Input: part model. Units: mm. Frame: model coordinates. Round coordinates to 2 decimals unless told otherwise and drop trailing zeros. Write each loop counter-clockwise with the first axis right and the second up, starting at its lowest first coordinate (ties: lowest second). Pieces come first, ordered by that corner, then holes. Notation, with made-up numbers: (27.5, 8.5) -> (35.5, 8.5) arc R17 cw to (35.5, 17.5) -> close; hole circle Ø9 at (39.25, 76.5). An arc over 180 degrees is marked (long way). Use CSV: the item, a comma, the result in double quotes.
```python
from build123d import *

# Parameters (mm, degrees)
SKETCH1_W           = 92.6
SKETCH1_H           = 300
BOSS_EXTRUDE1_DEPTH = 2
SKETCH2_R           = 2.25
SKETCH2_W           = 8.48
SKETCH2_H           = 51.5
SKETCH2_H_2         = 50
SKETCH2_H_3         = 53
CUT_EXTRUDE2_DEPTH  = 10
FILLET1_R           = 2
SKETCH3_R           = 1.85
CUT_EXTRUDE3_DEPTH  = 10
SKETCH4_R           = 1.85
SKETCH4_W           = 55.985713182
SKETCH4_H           = 38.778571429
CUT_EXTRUDE4_DEPTH  = 5
SKETCH5_R           = 1.85
SKETCH5_W           = 23.899789691
SKETCH5_H           = 32
CUT_EXTRUDE5_DEPTH  = 5


with BuildPart() as part:
    # Sketch1 → Boss-Extrude1 (new body)
    with BuildSketch(Plane.XY):
        Rectangle(SKETCH1_W, SKETCH1_H)
    extrude(amount=BOSS_EXTRUDE1_DEPTH)

    # Sketch2 → Cut-Extrude2 (cut)
    with BuildSketch(Plane.XY):
        with Locations((-42.06, 75)):
            Circle(SKETCH2_R)
        with Locations((42.06, 125)):
            Circle(SKETCH2_R)
        with Locations((42.06, 25)):
            Circle(SKETCH2_R)
        with Locations((42.06, -75)):
            Circle(SKETCH2_R)
        with Locations((-42.06, -25)):
            Circle(SKETCH2_R)
        with Locations((-42.06, -125)):
            Circle(SKETCH2_R)
        with Locations((-42.06, 124.25)):
            Rectangle(SKETCH2_W, SKETCH2_H)
        with Locations((42.06, 75)):
            Rectangle(SKETCH2_W, SKETCH2_H_2)
        with Locations((42.06, -25)):
            Rectangle(SKETCH2_W, SKETCH2_H_2)
        with Locations((-42.06, 25)):
            Rectangle(SKETCH2_W, SKETCH2_H_3)
        with Locations((-42.06, -75)):
            Rectangle(SKETCH2_W, SKETCH2_H_3)
        with Locations((42.06, -125)):
            Rectangle(SKETCH2_W, SKETCH2_H_2)
    extrude(amount=CUT_EXTRUDE2_DEPTH, mode=Mode.SUBTRACT)

    # Fillet1
    fillet1_edges = [part.edges().sort_by_distance(p)[0] for p in [
        (46.3, -100, 1),
        (37.82, -100, 1),
        (37.82, -150, 1),
        (46.3, 50, 1),
        (46.3, 100, 1),
        (37.82, 100, 1),
        (37.82, 50, 1),
        (-46.3, -48.5, 1),
        (-46.3, -101.5, 1),
        (-37.82, -101.5, 1),
        (-37.82, -48.5, 1),
        (37.82, 0, 1),
        (37.82, -50, 1),
        (46.3, -50, 1),
        (46.3, 0, 1),
        (46.3, 150, 1),
        (-46.3, 51.5, 1),
        (-46.3, -150, 1),
        (-46.3, -1.5, 1),
        (-37.82, -1.5, 1),
        (-37.82, 51.5, 1),
        (-46.3, 98.5, 1),
        (-37.82, 98.5, 1),
        (-37.82, 150, 1),
    ]]
    fillet(fillet1_edges, radius=FILLET1_R)

    # Sketch3 → Cut-Extrude3 (cut)
    with BuildSketch(Plane(origin=(0, 0, 0), x_dir=(-1, 0, 0), z_dir=(0, 0, -1))):
        with Locations((-25, -142)):
            Circle(SKETCH3_R)
        with Locations((25, -142)):
            Circle(SKETCH3_R)
        with Locations((-32, 142)):
            Circle(SKETCH3_R)
        with Locations((32, 142)):
            Circle(SKETCH3_R)
    extrude(amount=-CUT_EXTRUDE3_DEPTH, mode=Mode.SUBTRACT)

    # Sketch4 → Cut-Extrude4 (cut)
    with BuildSketch(Plane(origin=(0, 0, 0), x_dir=(-1, 0, 0), z_dir=(0, 0, -1))):
        with Locations((-32.95, -24.767949192)):
            Circle(SKETCH4_R)
        with Locations((0, -24.5)):
            Circle(SKETCH4_R)
        with Locations((32.95, -24.767949192)):
            Circle(SKETCH4_R)
        with Locations((-32.95, -69.732050808)):
            Circle(SKETCH4_R)
        with Locations((32.95, -69.732050808)):
            Circle(SKETCH4_R)
        with Locations((0.042856591, -49.889285715)):
            Rectangle(SKETCH4_W, SKETCH4_H)
    extrude(amount=-CUT_EXTRUDE4_DEPTH, mode=Mode.SUBTRACT)

    # Sketch5 → Cut-Extrude5 (cut)
    with BuildSketch(Plane(origin=(0, 0, 0), x_dir=(-1, 0, 0), z_dir=(0, 0, -1))):
        with Locations((-20, 100.5)):
            Circle(SKETCH5_R)
        with Locations((20, 100.5)):
            Circle(SKETCH5_R)
        with Locations((32, 37)):
            Circle(SKETCH5_R)
        with Locations((-32, 37)):
            Circle(SKETCH5_R)
        with Locations((-0.26347569, 103)):
            Rectangle(SKETCH5_W, SKETCH5_H)
    extrude(amount=-CUT_EXTRUDE5_DEPTH, mode=Mode.SUBTRACT)


solid = part.part
```
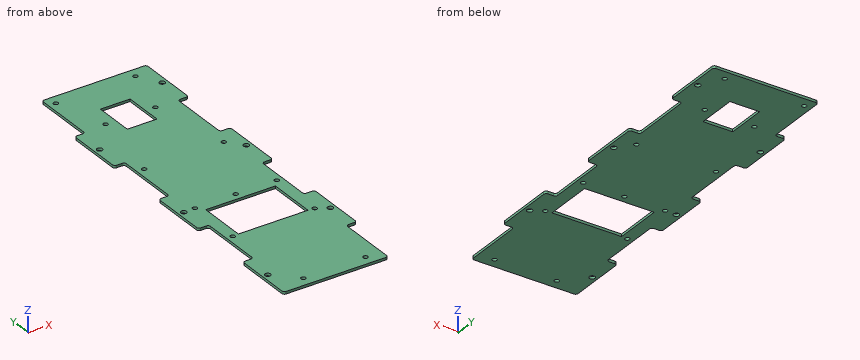
Item 1: Section query B-B on y = -94.5. Return the cut outline in (x, z).
Worked answers:
outline,"(-37.82, 0) -> (46.3, 0) -> (46.3, 2) -> (-37.82, 2) -> close"
Item 2: Line query: line 1 (Y direction, x = -7, z = 1.8); line 2 (Y direction, x = 20, z = 0.85); line 3 (Y direction, x = 42.06, z = 0.7). Output: solid intervals per line, ascending.
Worked answers:
line 1,"y = -150 to -69.28, -30.5 to 87, 119 to 150"
line 2,"y = -150 to -69.28, -30.5 to 98.65, 102.35 to 150"
line 3,"y = -100 to -77.25, -72.75 to -50, 0 to 22.75, 27.25 to 50, 100 to 122.75, 127.25 to 150"
Item 3: Section query A-A on x = -6.5. Return the cut outline in (y, z).
Worked answers:
outline,"(-150, 0) -> (-69.28, 0) -> (-69.28, 2) -> (-150, 2) -> close; (-30.5, 0) -> (87, 0) -> (87, 2) -> (-30.5, 2) -> close; (119, 0) -> (150, 0) -> (150, 2) -> (119, 2) -> close"
Item 4: Section query C-C on z = 1.3. Give the number of separate pieces and of enclosed holes in the cut face, plus the area to 3 significant figures.
Worked answers:
separate pieces,"1"
enclosed holes,"21"
area,"22,000 mm²"
Item 5: First-contact query: pin 1 Ø3 at (x, y) = (-32.95, -24.77) entering from +Z; pin 2 Ø1 at (x, z) = (-41, 1) entering from +Y; pin 3 Ø0.6 at (x, z) = (42.5, 0.5) entering from -Y. Flat tips, straight axial feed; report the tip coordinate or a pass-through.
Worked answers:
pin 1,"passes through"
pin 2,"stops at y = 98.5"
pin 3,"stops at y = -100"
